Check sheet for the modelled part. Datum: model origin and axes. Units: mm. Face numbers are marked on the shaded views. Round coordinates to 2 decimals unless told otherwise and drop trailing zeros. Loops run counter-clockwise (first coordinate to the right, second up) from the corner with the lowest first, then second, coordinate; pieces in that order, holes last. Notation, with made-up numbers: (58.5, 31.5) - (69.5, 31.5) arc R27 cw to (69.5, 52.5) - close; hole circle Ø11 at (74, -22). An arc over 180 degrees is marked (long way). Answer in a Markdown table with one row per item. Add a question column.
(1) Cross-section at C-C on z = -8.25. Enter the section's corners in (x, y).
(2) Cross-section at A-A on x = -11. Enter the section's corners in (y, z) (3 decimals), then the cut area to 3 significant figures.
(3) Cross-section at B-B on y = -2.75. Enter the section's corners in (x, z), then the cut area to 3 significant figures.
(4) Mould release check, pull along X, two halves, no side actions. Record for the marked faces 1 and 2: +X half, -X half, draft (parallel to the pull), parting line (faces both ways), or undercut.
(5) Gauge pin test, flat ends, axial feed: pin 1 (2 mm diameter, centred on x = -21, z = 1, fed in from -Y); pin 2 (10 mm diameter, centred on x = 19.5, z = 8.5, fed in from -Y); pin 3 (1.5 mm diameter, centred on x = -23.5, y = -1, fed in from -Z). Record the tip position at first contact, or that the pin passes through.
(6) Thickness scan on line 1 along Z through (x, y) = (-2, 1.5) (3 decimals); line 2 along X through (y, z) = (-2.5, -2); line 3 along Y through (x, z) = (20, 4.5). Record the ranges inside material, lowest first.
from build123d import *

# Parameters (mm, degrees)
SKETCH_1_W          = 2
SKETCH_1_H          = 13.69
EXTRUDE_1_DEPTH     = 1
EXTRUDE_START       = 1
SKETCH_1_3_R        = 4.499438526
SKETCH_1_3_R_2      = 3
SKETCH_1_3_W        = 4.417890806
SKETCH_1_3_H        = 1
SKETCH_1_3_W_2      = 11.749439362
SKETCH_1_3_H_2      = 0.999974731
EXTRUDE_2_DEPTH     = 1.5
FILLET_1_R          = 1
SKETCH_1_4_R        = 3
EXTRUDE_3_DEPTH     = 4
SKETCH_4_R          = 1.65
CUT_EXTRUDE_1_DEPTH = 2.5
FILLET_2_R          = 1.5
FILLET_3_R          = 10
SKETCH_9_R          = 3
EXTRUDE_6_DEPTH     = 4
SKETCH_10_R         = 2
CUT_EXTRUDE_3_DEPTH = 2.5
FILLET_5_R          = 1.5


with BuildPart() as part:
    # 草图1 → 凸台-拉伸1 (new body)
    with BuildSketch(Plane(origin=(0, 0, 0), x_dir=(1, 0, 0), z_dir=(0, 1, 0))):
        with BuildLine():
            Line((18.474806794, -10.844974731), (28.247830948, -3.308032201))
            ThreePointArc((28.247830948, -3.308032201), (29.998869582, 0.33088638), (28.126002395, 3.908627739))
            Line((28.126002395, 3.908627739), (18.474816537, 10.845))
            Line((18.474816537, 10.845), (-18.474816537, 10.845))
            Line((-18.474816537, 10.845), (-28.126002395, 3.908627739))
            ThreePointArc((-28.126002395, 3.908627739), (-29.998869582, 0.330886398), (-28.247830977, -3.308032179))
            Line((-28.247830977, -3.308032179), (-18.474806794, -10.844974731))
            Line((-18.474806794, -10.844974731), (18.474806794, -10.844974731))
        make_face()
        with Locations((-19.29, 0)):
            Rectangle(SKETCH_1_W, SKETCH_1_H, mode=Mode.SUBTRACT)
    extrude(amount=EXTRUDE_1_DEPTH)

    # 草图1<3> → 凸台-拉伸2 (add)
    # profile 1 of 10: a face of its own
    with BuildSketch(Plane(origin=(0, 0, 0), x_dir=(1, 0, 0), z_dir=(0, 1, 0)).offset(EXTRUDE_START)):
        with Locations((-25.50007206, 0.254939612)):
            Circle(SKETCH_1_3_R)
        with Locations((-25.50007206, 0.254939612)):
            Circle(SKETCH_1_3_R_2, mode=Mode.SUBTRACT)
    # profile 2 of 10: a face of its own
    with BuildSketch(Plane(origin=(0, 0, 0), x_dir=(1, 0, 0), z_dir=(0, 1, 0)).offset(EXTRUDE_START)):
        with Locations((-25.50007206, 0.254939612)):
            Circle(SKETCH_1_3_R_2)
    # profile 3 of 10: a face of its own
    with BuildSketch(Plane(origin=(0, 0, 0), x_dir=(1, 0, 0), z_dir=(0, 1, 0)).offset(EXTRUDE_START)):
        with BuildLine():
            Line((-19.79, 6.845), (-19.79, 9.89976879))
            Line((-19.79, 9.89976879), (-28.126002395, 3.908627739))
            ThreePointArc((-28.126002395, 3.908627739), (-23.44705782, 4.258697795), (-21.000633534, 0.254939612))
            ThreePointArc((-21.000633534, 0.254939612), (-23.514930413, -3.782901357), (-28.247830977, -3.308032179))
            Line((-28.247830977, -3.308032179), (-19.79, -9.830699574))
            Line((-19.79, -9.830699574), (-19.79, -6.845))
            Line((-19.79, -6.845), (-20.29, -6.845))
            Line((-20.29, -6.845), (-20.29, 6.845))
            Line((-20.29, 6.845), (-19.79, 6.845))
        make_face()
    # profile 4 of 10: a face of its own
    with BuildSketch(Plane(origin=(0, 0, 0), x_dir=(1, 0, 0), z_dir=(0, 1, 0)).offset(EXTRUDE_START)):
        with BuildLine():
            Line((-18.474816537, 10.845), (-19.79, 9.89976879))
            Line((-19.79, 9.89976879), (-19.79, 6.845))
            Line((-19.79, 6.845), (-18.29, 6.845))
            Line((-18.29, 6.845), (-18.29, 7.045))
            ThreePointArc((-18.29, 7.045), (-17.469898987, 9.024898987), (-15.49, 9.845))
            Line((-15.49, 9.845), (-4.417890806, 9.845))
            Line((-4.417890806, 9.845), (-4.417890806, 10.845))
            Line((-4.417890806, 10.845), (-18.474816537, 10.845))
        make_face()
    # profile 5 of 10: a face of its own
    with BuildSketch(Plane(origin=(0, 0, 0), x_dir=(1, 0, 0), z_dir=(0, 1, 0)).offset(EXTRUDE_START)):
        with Locations((-2.208945403, 10.345)):
            Rectangle(SKETCH_1_3_W, SKETCH_1_3_H)
    # profile 6 of 10: a face of its own
    with BuildSketch(Plane(origin=(0, 0, 0), x_dir=(1, 0, 0), z_dir=(0, 1, 0)).offset(EXTRUDE_START)):
        with BuildLine():
            Line((-19.79, -6.845), (-19.79, -9.830699574))
            Line((-19.79, -9.830699574), (-18.474806794, -10.844974731))
            Line((-18.474806794, -10.844974731), (-11.749439362, -10.844974731))
            Line((-11.749439362, -10.844974731), (-11.749439362, -9.845))
            Line((-11.749439362, -9.845), (-15.49, -9.845))
            ThreePointArc((-15.49, -9.845), (-17.469898987, -9.024898987), (-18.29, -7.045))
            Line((-18.29, -7.045), (-18.29, -6.845))
            Line((-18.29, -6.845), (-19.79, -6.845))
        make_face()
    # profile 7 of 10: a face of its own
    with BuildSketch(Plane(origin=(0, 0, 0), x_dir=(1, 0, 0), z_dir=(0, 1, 0)).offset(EXTRUDE_START)):
        with Locations((-5.874719681, -10.344987365)):
            Rectangle(SKETCH_1_3_W_2, SKETCH_1_3_H_2)
    # profile 8 of 10: a face of its own
    with BuildSketch(Plane(origin=(0, 0, 0), x_dir=(1, 0, 0), z_dir=(0, 1, 0)).offset(EXTRUDE_START)):
        with BuildLine():
            Line((18.474816537, 10.845), (0, 10.845))
            Line((0, 10.845), (0, 9.845))
            Line((0, 9.845), (15.49, 9.845))
            ThreePointArc((15.49, 9.845), (17.469898987, 9.024898987), (18.29, 7.045))
            Line((18.29, 7.045), (18.29, -7.045))
            ThreePointArc((18.29, -7.045), (17.469898987, -9.024898987), (15.49, -9.845))
            Line((15.49, -9.845), (0, -9.845))
            Line((0, -9.845), (0, -10.844974731))
            Line((0, -10.844974731), (18.474806794, -10.844974731))
            Line((18.474806794, -10.844974731), (19.79, -9.830699574))
            Line((19.79, -9.830699574), (19.79, 9.89976879))
            Line((19.79, 9.89976879), (18.474816537, 10.845))
        make_face()
    # profile 9 of 10: a face of its own
    with BuildSketch(Plane(origin=(0, 0, 0), x_dir=(1, 0, 0), z_dir=(0, 1, 0)).offset(EXTRUDE_START)):
        with BuildLine():
            Line((28.126002395, 3.908627739), (19.79, 9.89976879))
            Line((19.79, 9.89976879), (19.79, -9.830699574))
            Line((19.79, -9.830699574), (28.247830948, -3.308032201))
            ThreePointArc((28.247830948, -3.308032201), (21.001274538, 0.178992845), (28.126002395, 3.908627739))
        make_face()
    # profile 10 of 10: a face of its own
    with BuildSketch(Plane(origin=(0, 0, 0), x_dir=(1, 0, 0), z_dir=(0, 1, 0)).offset(EXTRUDE_START)):
        with Locations((25.50007206, 0.254939612)):
            Circle(SKETCH_1_3_R)
    extrude(amount=EXTRUDE_2_DEPTH)

    # 圆角1
    fillet_1_edges = [part.edges().sort_by_distance(p)[0] for p in [
        (-20.29, 1.25, -6.845),
        (-20.29, 1.25, 6.845),
    ]]
    fillet(fillet_1_edges, radius=FILLET_1_R)

    # 草图1<4> → 凸台-拉伸3 (add)
    with BuildSketch(Plane(origin=(0, 0, 0), x_dir=(1, 0, 0), z_dir=(0, 1, 0))):
        with Locations(Location((-25.50007206, 0.254939612, 0), (0, 0, 270))):
            Circle(SKETCH_1_4_R)
    extrude(amount=-EXTRUDE_3_DEPTH)

    # 草图4 → 切除-拉伸1 (cut)
    with BuildSketch(Plane.XZ.offset(4)):
        with Locations(Location((-25.50007206, -0.254939612, 0), (0, 0, 270))):
            Circle(SKETCH_4_R)
        with Locations((25.5, -0.255)):
            Circle(SKETCH_4_R)
    extrude(amount=-CUT_EXTRUDE_1_DEPTH, mode=Mode.SUBTRACT)

    # 圆角2
    fillet_2_edges = [part.edges().sort_by_distance(p)[0] for p in [
        (-25.50007206, 0, -3.254939612),
    ]]
    fillet(fillet_2_edges, radius=FILLET_2_R)

    # 圆角3
    fillet_3_edges = [part.edges().sort_by_distance(p)[0] for p in [
        (-18.474806794, 1.25, 10.844974731),
        (-18.474816537, 1.25, -10.845),
        (18.474816537, 1.25, -10.845),
        (18.474806794, 1.25, 10.844974731),
    ]]
    fillet(fillet_3_edges, radius=FILLET_3_R)

    # 草图9 → 凸台-拉伸6 (add)
    with BuildSketch(Plane.XZ):
        with Locations(Location((25.50007206, -0.254939612, 0), (0, 0, 90))):
            Circle(SKETCH_9_R)
    extrude(amount=EXTRUDE_6_DEPTH)

    # 草图10 → 切除-拉伸3 (cut)
    with BuildSketch(Plane.XZ.offset(4)):
        with Locations(Location((25.50007206, -0.254939612, 0), (0, 0, 270))):
            Circle(SKETCH_10_R)
    extrude(amount=-CUT_EXTRUDE_3_DEPTH, mode=Mode.SUBTRACT)

    # 圆角5
    fillet_5_edges = [part.edges().sort_by_distance(p)[0] for p in [
        (25.50007206, 0, -3.254939612),
    ]]
    fillet(fillet_5_edges, radius=FILLET_5_R)


solid = part.part
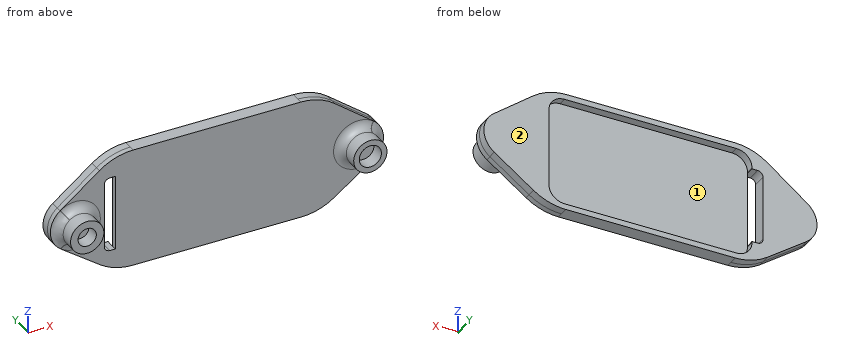
Answers:
| question | item | result |
|---|---|---|
| 1 | outline | (-22.09, 0) - (22.09, 0) - (22.09, 2.5) - (18.02, 2.5) - (18.02, 1) - (-18.02, 1) - (-18.02, 2.5) - (-22.09, 2.5) - close |
| 2 | outline | (0, -10.845) - (2.5, -10.845) - (2.5, -9.845) - (1, -9.845) - (1, 9.845) - (2.5, 9.845) - (2.5, 10.845) - (0, 10.845) - close |
| 2 | area | 24.7 mm^2 |
| 3 | outline | circle Ø6 at (-25.5, -0.25); circle Ø6 at (25.5, -0.25); hole circle Ø3.3 at (-25.5, -0.25); hole circle Ø4 at (25.5, -0.25) |
| 3 | area | 35.4 mm^2 |
| 4 | face 1 | undercut |
| 4 | face 2 | draft |
| 5 | pin 1 | stops at y = -0.25 |
| 5 | pin 2 | stops at y = 0 |
| 5 | pin 3 | stops at z = -3.41 |
| 6 | line 1 | z = -10.845 to -9.845, 9.845 to 10.845 |
| 6 | line 2 | x = -27.94 to -23.06, 23.06 to 24.52, 26.48 to 27.94 |
| 6 | line 3 | y = 0 to 2.5 |
